Design review of the part built by this model. Coordinates are the model's own, in mm. Give positions to 0.01 mm unless a question says otherwise; leave off trailing zeros. Loops run counter-clockwise (first coordinate to the right, second up) from the corner with the lowest first, then second, coordinate; pieces in that order, holes last. Notation, with made-up numbers: M 66,78.5 L 76,78.5 A16 cw 76,88.5 Z; hole C -35.75,88 d5. An arc over 180 degrees is marked long. Use a Markdown table: item, result. Add a question column.
(1) For probe 1 along Y at (x, z) = (-0.1, -2); probe 2 along Y at (x, z) = (0.3, -9); probe 3 along Z at (x, y) = (0.2, 0), list the stretches that pass through material, from the lowest coordinate up.
(2) Add section A-A, the plane y = -0.5. Give the boundary of the cut face in (x, z) (1 decimal).
(3) Add section B-B, the plane x = 0.25. Give the boundary of the cut face in (y, z), then the cut area to 3 significant figures.
(4) Insertion check: pin 1 Ø1.2 at (y, z) = (15.5, -2) entering from -X. The pin has a flat end and moves straight along its axis. Give the tip position at first contact, or say it passes through.
```python
from build123d import *

# Parameters (mm, degrees)
SKETCH3_R                = 0.9906
BOSS_EXTRUDE1_DEPTH      = 0.635
BOSS_EXTRUDE1_DEPTH_BACK = 0.635
FILLET1_R                = 1.3589


with BuildPart() as part:
    # Sketch3 → Boss-Extrude1 (new body, two sides)
    with BuildSketch(Plane(origin=(0, 0, 0), x_dir=(0, 0, -1), z_dir=(1, 0, 0))) as boss_extrude1_sk:
        with BuildLine():
            Line((-3.777983958, 17.78027311), (-6.047809043, 13.75309371))
            ThreePointArc((-6.047809043, 13.75309371), (0, -16.4719), (6.047809043, 13.75309371))
            Line((6.047809043, 13.75309371), (3.777983958, 17.78027311))
            Line((3.777983958, 17.78027311), (0.311412014, 17.840782349))
            Line((0.311412014, 17.840782349), (0.23073303, 13.218686423))
            ThreePointArc((0.23073303, 13.218686423), (0, -13.2207), (-0.23073303, 13.218686423))
            Line((-0.23073303, 13.218686423), (-0.311412014, 17.840782349))
            Line((-0.311412014, 17.840782349), (-3.777983958, 17.78027311))
        make_face()
        with Locations((-2.004358494, 15.499479767)):
            Circle(SKETCH3_R, mode=Mode.SUBTRACT)
        with Locations((2.004358494, 15.499479767)):
            Circle(SKETCH3_R, mode=Mode.SUBTRACT)
    extrude(amount=BOSS_EXTRUDE1_DEPTH)
    extrude(boss_extrude1_sk.sketch, amount=-BOSS_EXTRUDE1_DEPTH_BACK)

    # Fillet1
    fillet1_edges = [part.edges().sort_by_distance(p)[0] for p in [
        (0, 13.75309371, 6.047809043),
        (0, 17.78027311, 3.777983958),
        (0, 13.218686423, 0.23073303),
        (0, 13.218686423, -0.23073303),
        (0, 17.78027311, -3.777983958),
        (0, 13.75309371, -6.047809043),
    ]]
    fillet(fillet1_edges, radius=FILLET1_R)


solid = part.part
```
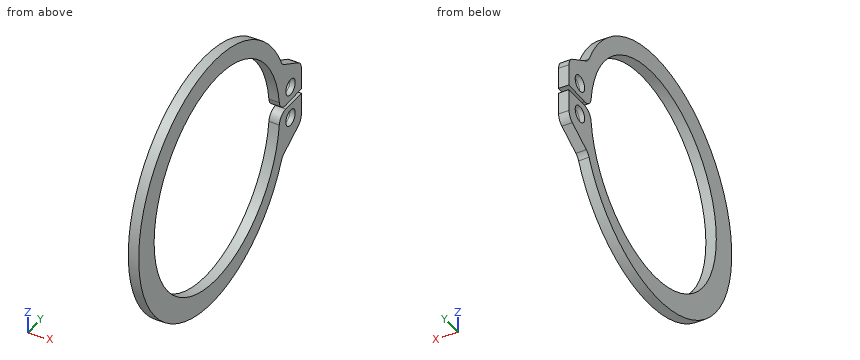
Established:
| question | item | result |
|---|---|---|
| 1 | probe 1 | -16.34 to -13.07, 13.07 to 14.51, 16.49 to 17.81 |
| 1 | probe 2 | -13.64 to -9.68, 9.68 to 12.13 |
| 1 | probe 3 | -15.7 to -13.22, 13.22 to 15.7 |
| 2 | outline | M -0.6,-15.7 L 0.6,-15.7 L 0.6,-13.2 L -0.6,-13.2 Z; M -0.6,13.2 L 0.6,13.2 L 0.6,15.7 L -0.6,15.7 Z |
| 3 | outline | M 13.14,-1.46 A13.22 cw long 13.14,1.46 A1.36 ccw 14.51,0.25 L 17.84,0.31 L 17.79,3 A1.36 ccw 17.1,4.16 L 14.15,5.82 A1.36 cw 13.58,6.45 A15.72 ccw long 13.58,-6.45 A1.36 cw 14.15,-5.82 L 17.1,-4.16 A1.36 ccw 17.79,-3 L 17.84,-0.31 L 14.51,-0.25 A1.36 ccw Z; hole C 15.5,-2 d1.98; hole C 15.5,2 d1.98 |
| 3 | area | 247 mm^2 |
| 4 | pin 1 | through |
